Here's how the part is built. I have some questions about the finished solid (model axes, mm). Face numbers are marked on the shaded views. A direction names the side the tool comes from. Round coordinates to 2 decimals unless told otherwise and drop trailing zeros. Loops run counter-clockwise (first coordinate to the right, second up) from the corner with the lowest first, then second, coordinate; pieces in that order, holes last. Notation, with made-up numbers: (-7, 14.5) -> (52, 14.5) arc R21 cw to (52, 27.5) -> close; hole circle Ø3 at (-20, 72.5). An arc over 180 degrees is marked (long way). Use one line per item in the form item = value. Start each with the question number.
Item 1: Thinking about a two-plate mould opening in Y: for the marked faces 3, 4, 5 and 6, which applies, released by +Y, released by -Y, zero draft, split by the parting line, or undercut?
Item 2: I'm going to push flat-ended pins straight in: pin 1 Ø10 at (x, y) = (-14.5, -1.5) entering from -Z; pin 2 Ø2 at (x, z) = (7, -21) entering from +Y; pin 3 Ø6 at (x, y) = (-12.5, 15.5) entering from -Z; pin 4 Ø3 at (y, z) = (10, -13.5) entering from +X. Where does each tip first touch, or does it pass through?
Item 3: If I drill on L1, parallel to Y at x = 0, z = -19.5; L2, parallel to X at y = 5, z = 6.5 (3 decimals); L3, parallel to Y at x = 6, z = -12.5, over which ranges is the centre line in solid material (lowest first)? Write a range as [from, to].
Item 4: If we section it at D-D (y = -6): Write out the boundary of the cut face in (x, z).
Item 5: If we section it at C-C (z = 7.5): Write out the boundary of the cut face in (x, y).
Item 6: If we section it at B-B (y = 0): Write out the boundary of the cut face in (x, z).
Item 7: If we section it at A-A (x = 0): Write out the boundary of the cut face in (y, z), then the cut area to 3 significant figures.
Item 8: For the marked faces 1 and 2, which set-ups out of +Z, -Z, +X, -X, +Y, -Y let a thin tool reach every point of the face, with its end or its side?
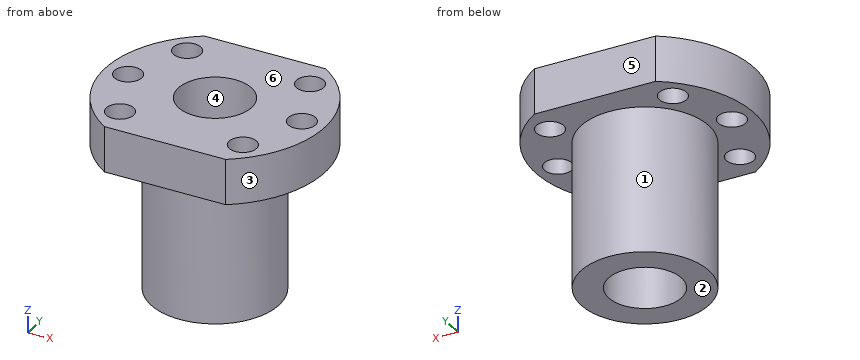
```python
from build123d import *

# Parameters (mm, degrees)
SKETCH1_R           = 3
SKETCH1_R_2         = 14
SKETCH1_R_3         = 8
BOSS_EXTRUDE1_DEPTH = 10
BOSS_EXTRUDE2_START = -32
SKETCH1_3_R         = 14
SKETCH1_3_R_2       = 8
BOSS_EXTRUDE2_DEPTH = 32


with BuildPart() as part:
    # Sketch1 → Boss-Extrude1 (new body)
    # profile 1 of 2: a face of its own
    with BuildSketch(Plane.XY):
        with BuildLine():
            Line((-13.266499161, 20), (13.266499161, 20))
            ThreePointArc((13.266499161, 20), (24, 0), (13.266499161, -20))
            Line((13.266499161, -20), (-13.266499161, -20))
            ThreePointArc((-13.266499161, -20), (-24, 0), (-13.266499161, 20))
        make_face()
        with Locations((13.435028843, 13.435028843)):
            Circle(SKETCH1_R, mode=Mode.SUBTRACT)
        with Locations((-13.435028843, 13.435028843)):
            Circle(SKETCH1_R, mode=Mode.SUBTRACT)
        with Locations((-19, 0)):
            Circle(SKETCH1_R, mode=Mode.SUBTRACT)
        with Locations((-13.435028843, -13.435028843)):
            Circle(SKETCH1_R, mode=Mode.SUBTRACT)
        with Locations((13.435028843, -13.435028843)):
            Circle(SKETCH1_R, mode=Mode.SUBTRACT)
        with Locations((19, 0)):
            Circle(SKETCH1_R, mode=Mode.SUBTRACT)
        Circle(SKETCH1_R_2, mode=Mode.SUBTRACT)
    # profile 2 of 2: a face of its own
    with BuildSketch(Plane.XY):
        Circle(SKETCH1_R_2)
        Circle(SKETCH1_R_3, mode=Mode.SUBTRACT)
    extrude(amount=BOSS_EXTRUDE1_DEPTH)

    # Sketch1<3> → Boss-Extrude2 (add)
    with BuildSketch(Plane.XY.offset(BOSS_EXTRUDE2_START)):
        Circle(SKETCH1_3_R)
        Circle(SKETCH1_3_R_2, mode=Mode.SUBTRACT)
    extrude(amount=BOSS_EXTRUDE2_DEPTH)


solid = part.part
```
Values found:
q1.face_3 = split by the parting line
q1.face_4 = undercut
q1.face_5 = released by +Y
q1.face_6 = zero draft
q2.pin_1 = -32
q2.pin_2 = 12.65
q2.pin_3 = 0
q2.pin_4 = 11.12
q3.L1 = [-14, -8], [8, 14]
q3.L2 = [-23.473, -6.245], [6.245, 23.473]
q3.L3 = [-12.65, -5.29], [5.29, 12.65]
q4.outline = (-23.24, 0) -> (-12.65, 0) -> (-12.65, -32) -> (-5.29, -32) -> (-5.29, 10) -> (-23.24, 10) -> close; (5.29, -32) -> (12.65, -32) -> (12.65, 0) -> (23.24, 0) -> (23.24, 10) -> (5.29, 10) -> close
q5.outline = (-13.27, -20) -> (13.27, -20) arc R24 ccw to (13.27, 20) -> (-13.27, 20) arc R24 ccw to start; hole circle Ø6 at (-19, 0); hole circle Ø6 at (-13.44, -13.44); hole circle Ø6 at (-13.44, 13.44); hole circle Ø16 at (0, 0); hole circle Ø6 at (13.44, -13.44); hole circle Ø6 at (13.44, 13.44); hole circle Ø6 at (19, 0)
q6.outline = (-24, 0) -> (-22, 0) -> (-22, 10) -> (-24, 10) -> close; (-16, 0) -> (-14, 0) -> (-14, -32) -> (-8, -32) -> (-8, 10) -> (-16, 10) -> close; (8, -32) -> (14, -32) -> (14, 0) -> (16, 0) -> (16, 10) -> (8, 10) -> close; (22, 0) -> (24, 0) -> (24, 10) -> (22, 10) -> close
q7.outline = (-20, 0) -> (-14, 0) -> (-14, -32) -> (-8, -32) -> (-8, 10) -> (-20, 10) -> close; (8, -32) -> (14, -32) -> (14, 0) -> (20, 0) -> (20, 10) -> (8, 10) -> close
q7.area = 624 mm2
q8.face_1 = -Z
q8.face_2 = -Z, +X, -X, +Y, -Y
